from build123d import *

# Parameters (mm, degrees)
SKETCH1_R           = 3.5
BOSS_EXTRUDE1_DEPTH = 1.2
BOSS_EXTRUDE2_DEPTH = 2.4


with BuildPart() as part:
    # Sketch1 → Boss-Extrude1 (new body)
    with BuildSketch(Plane(origin=(0, 0, 0), x_dir=(1, 0, 0), z_dir=(0, 1, 0))):
        Polygon((-60, -40), (-35, -40), (-35, -140), (35, -140), (35, -40), (60, -40), (60, 40), (-60, 40), align=None)
        with Locations(Location((0, -125, 0), (0, 0, 270))):
            Circle(SKETCH1_R, mode=Mode.SUBTRACT)
    extrude(amount=BOSS_EXTRUDE1_DEPTH)

    # Sketch2 → Boss-Extrude2 (add)
    with BuildSketch(Plane(origin=(0, 1.2, 0), x_dir=(1, 0, 0), z_dir=(0, 1, 0))):
        Polygon((-60, -40), (-35, -40), (-35, -140), (35, -140), (35, -40), (60, -40), (60, 0), (60, 40), (-60, 40), (-60, 0), align=None)
        Polygon((-55, -35), (-30, -35), (-30, -135), (30, -135), (30, -35), (55, -35), (55, 0), (55, 35), (-55, 35), (-55, 0), align=None, mode=Mode.SUBTRACT)
    extrude(amount=BOSS_EXTRUDE2_DEPTH)


solid = part.part
Verification items for the finished model (mm, model axes). A direction names the side the tool comes from. Coordinates: 2 decimals unless noted, no trailing zeros. Order: outer loops, then holes, each group sorted by start corner. A loop starts at its lowest first (then second) coordinate and runs counter-clockwise, first axis right, second up. Notation, with made-up numbers: M 28,20.5 L 42,20.5 A9 ccw 42,30.5 Z; hole C 7.25,37 d11. An arc over 180 degrees is marked long. One line per item, written item: value. Start each with the question number.
Item 1: Sectioned sample at A-A (x = 0). Enter the section's corners in (y, z), then the cut area to 3 significant figures.
Item 2: Sectioned sample at D-D (x = 20). Enter the section's corners in (y, z), then the cut area to 3 significant figures.
Item 3: Gauge pin test, flat ends, axial feed: pin 1 (8 mm diameter, centred on x = 0, z = 125, fed in from +Y); pin 2 (0.7 mm diameter, centred on y = 2.5, z = 79.5, fed in from -X); pin 3 (1.8 mm diameter, centred on x = -46, y = 1, fed in from +Z); pin 4 (12 mm diameter, centred on x = 42.5, z = 75, fed in from -Y). Record the tip position at first contact, or that the pin passes through.
Item 4: Scan lines: probe 1 along X at (y, z) = (3.4, 67); probe 2 along X at (y, z) = (2.5, 38.5); probe 3 along Z at (x, y) = (33, 1.3). Record each from-to range of solid material in increasing order.
Item 5: Sectioned sample at B-B (z = 125). Enter the section's corners in (x, y), then the cut area to 3 significant figures.
Item 6: Access from +Z, -Z, +X, -X, +Y, -Y to the whole of each face (thin tool, end or side, straight path). Record for faces 5 (the flat face through (-31, 3.6, 36)), 6 (the flat face through (35, 2, 91)), 7 (the flat face through (-48, 2, 40)).
Item 7: Sectioned sample at C-C (y = 1.85). Enter the section's corners in (x, z), then the cut area to 3 significant figures.
Item 8: Mould release check, pull along X, two halves, no side actions. Record for faces 1 (the cylindrical face through (1.05, 0.59, 128.34)), 2 (the flat face through (60, 2, 1)), 3 (the flat face through (-1, 1.2, 30)), 4 (the flat face through (1, 2, -40)): released by +X, released by -X, zero draft, split by the parting line, or undercut.
Conclusion:
1. outline: M 0,-40 L 3.6,-40 L 3.6,-35 L 1.2,-35 L 1.2,121.5 L 0,121.5 Z; M 0,128.5 L 1.2,128.5 L 1.2,135 L 3.6,135 L 3.6,140 L 0,140 Z
1. area: 232 mm^2
2. outline: M 0,-40 L 3.6,-40 L 3.6,-35 L 1.2,-35 L 1.2,135 L 3.6,135 L 3.6,140 L 0,140 Z
2. area: 240 mm^2
3. pin 1: stops at y = 1.2
3. pin 2: stops at x = -35
3. pin 3: stops at z = 40
3. pin 4: passes through
4. probe 1: x = -35 to -30, 30 to 35
4. probe 2: x = -60 to -30, 30 to 60
4. probe 3: z = -40 to -35, 35 to 140
5. outline: M -35,0 L -3.5,0 L -3.5,1.2 L -30,1.2 L -30,3.6 L -35,3.6 Z; M 3.5,0 L 35,0 L 35,3.6 L 30,3.6 L 30,1.2 L 3.5,1.2 Z
5. area: 99.6 mm^2
6. face 5: +Z, -Z, +X, -X, +Y
6. face 6: +Z, +X, +Y, -Y
6. face 7: +Z, -X, +Y, -Y
7. outline: M -60,-40 L 60,-40 L 60,40 L 35,40 L 35,140 L -35,140 L -35,40 L -60,40 Z; hole M -55,-35 L 55,-35 L 55,35 L 30,35 L 30,135 L -30,135 L -30,35 L -55,35 Z
7. area: 2,900 mm^2
8. face 1: undercut
8. face 2: released by +X
8. face 3: undercut
8. face 4: zero draft
